Read the model definition and answer for the solid it produces. Units are mm, in the model's axes. A direction names the side the tool comes from. Round coordinates to 2 decimals unless told otherwise and drop trailing zeros. Order: outer loops, then holes, each group sorted by start corner. A loop starts at its lowest first (then second) coordinate and runs counter-clockwise, first axis right, second up. Notation, with made-up numbers: (-14.5, -36.5) - (0.5, -36.5) arc R14 ccw to (0.5, -31.5) - close; hole circle Ø7 at (14, 38.25). An arc over 180 degrees is marked (long way). One line per question, with ' | ' between items. Start each with the question number.
1) The part is cut by section A-A, the plane x = -3.5. Give the vertices of the cut face in (y, z).
2) The mould has two halves that part along X. Classify faces 4 (the flat face through (-2, -13.7, 1)), 5 (the flat face through (-7.5, 19, 2)), 6 (the cylindrical face through (-1.216, 1.115, 2.465)): pulls with the +X half, pulls with the -X half, needs draft (parallel to the pull), parting line crosses it, or undercut.
3) For faces 1 (the flat face through (-2, 13.7, 1)), 2 (the cylindrical face through (6.65, 14.93, 3.73)), 3 (the flat face through (-7.5, 0, 2)), determine the directions among +Z, -Z, +X, -X, +Y, -Y from which every point of the face is accessible in a straight line to the end or side of a thin tool.
4) The part is cut by section B-B, the plane z = 3.9. Give the vertices of the cut face in (x, y), plus the area to 3 significant figures.
5) The part is cut by section C-C, the plane x = 0. Give the vertices of the cut face in (y, z), plus the area to 3 significant figures.
6) The part is cut by section D-D, the plane y = -12.5. Give the vertices of the cut face in (x, z).
7) Straight lines are drawn through the part: line 1 (Y direction, x = 0, z = 2.9); line 2 (Y direction, x = -3, z = 1.45); line 3 (Y direction, x = -4.75, z = 2.8). For each, find the intervals that lie inside material, in ascending order. Write a range as from..to.
from build123d import *

# Parameters (mm, degrees)
SKETCH1_R           = 1.65
BOSS_EXTRUDE1_DEPTH = 5
CUT_EXTRUDE1_START  = -2.5
CUT_EXTRUDE1_DEPTH  = 2.5


with BuildPart() as part:
    # Sketch1 → Boss-Extrude1 (new body)
    with BuildSketch(Plane.XY):
        with BuildLine():
            Line((-7.5, 16.7), (3, 16.7))
            ThreePointArc((3, 16.7), (4.5, 15.2), (3, 13.7))
            Line((3, 13.7), (-7.5, 13.7))
            Line((-7.5, 13.7), (-7.5, -13.7))
            Line((-7.5, -13.7), (3, -13.7))
            ThreePointArc((3, -13.7), (4.5, -15.2), (3, -16.7))
            Line((3, -16.7), (-7.5, -16.7))
            Line((-7.5, -16.7), (-7.5, -20))
            Line((-7.5, -20), (4.5, -20))
            ThreePointArc((4.5, -20), (6.621320344, -19.121320344), (7.5, -17))
            Line((7.5, -17), (7.5, 17))
            ThreePointArc((7.5, 17), (6.621320344, 19.121320344), (4.5, 20))
            Line((4.5, 20), (-7.5, 20))
            Line((-7.5, 20), (-7.5, 16.7))
        make_face()
        Circle(SKETCH1_R, mode=Mode.SUBTRACT)
    extrude(amount=BOSS_EXTRUDE1_DEPTH)

    # Sketch2 → Cut-Extrude1 (cut)
    with BuildSketch(Plane.XY.offset(5).offset(CUT_EXTRUDE1_START)):
        with BuildLine():
            Line((3.4, -11.75), (-7.5, -11.75))
            Line((-7.5, -11.75), (-7.5, -13.7))
            Line((-7.5, -13.7), (3, -13.7))
            ThreePointArc((3, -13.7), (4.5, -15.2), (3, -16.7))
            Line((3, -16.7), (-7.5, -16.7))
            Line((-7.5, -16.7), (-7.5, -18.25))
            Line((-7.5, -18.25), (3.4, -18.25))
            ThreePointArc((3.4, -18.25), (6.65, -15), (3.4, -11.75))
        make_face()
        with BuildLine():
            Line((3.4, 18.25), (-7.5, 18.25))
            Line((-7.5, 18.25), (-7.5, 16.7))
            Line((-7.5, 16.7), (3, 16.7))
            ThreePointArc((3, 16.7), (4.5, 15.2), (3, 13.7))
            Line((3, 13.7), (-7.5, 13.7))
            Line((-7.5, 13.7), (-7.5, 11.75))
            Line((-7.5, 11.75), (3.4, 11.75))
            ThreePointArc((3.4, 11.75), (6.65, 15), (3.4, 18.25))
        make_face()
    extrude(amount=CUT_EXTRUDE1_DEPTH, mode=Mode.SUBTRACT)


solid = part.part
Values:
1) outline: (-20, 0) - (-16.7, 0) - (-16.7, 2.5) - (-18.25, 2.5) - (-18.25, 5) - (-20, 5) - close; (-13.7, 0) - (13.7, 0) - (13.7, 2.5) - (11.75, 2.5) - (11.75, 5) - (-11.75, 5) - (-11.75, 2.5) - (-13.7, 2.5) - close; (16.7, 0) - (20, 0) - (20, 5) - (18.25, 5) - (18.25, 2.5) - (16.7, 2.5) - close
2) face 4: needs draft | face 5: pulls with the -X half | face 6: undercut
3) face 1: +Z, -Z, -X | face 2: +Z, -X | face 3: +Z, -Z, -X, +Y, -Y
4) outline: (-7.5, -20) - (4.5, -20) arc R3 ccw to (7.5, -17) - (7.5, 17) arc R3 ccw to (4.5, 20) - (-7.5, 20) - (-7.5, 18.25) - (3.4, 18.25) arc R3.25 cw to (3.4, 11.75) - (-7.5, 11.75) - (-7.5, -11.75) - (3.4, -11.75) arc R3.25 cw to (3.4, -18.25) - (-7.5, -18.25) - close; hole circle Ø3.3 at (0, 0) | area: 413 mm^2
5) outline: (-20, 0) - (-16.7, 0) - (-16.7, 2.5) - (-18.25, 2.5) - (-18.25, 5) - (-20, 5) - close; (-13.7, 0) - (-1.65, 0) - (-1.65, 5) - (-11.75, 5) - (-11.75, 2.5) - (-13.7, 2.5) - close; (1.65, 0) - (13.7, 0) - (13.7, 2.5) - (11.75, 2.5) - (11.75, 5) - (1.65, 5) - close; (16.7, 0) - (20, 0) - (20, 5) - (18.25, 5) - (18.25, 2.5) - (16.7, 2.5) - close | area: 136 mm^2
6) outline: (-7.5, 0) - (7.5, 0) - (7.5, 5) - (5.48, 5) - (5.48, 2.5) - (-7.5, 2.5) - close
7) line 1: y = -20..-18.25, -11.75..-1.65, 1.65..11.75, 18.25..20 | line 2: y = -20..-16.7, -13.7..13.7, 16.7..20 | line 3: y = -20..-18.25, -11.75..11.75, 18.25..20
